Work out the finished part from the listing and answer in its coordinate system (mm). Face numbers are marked on the shaded views. A direction names the side the tool comes from. Give positions to 0.01 mm unless a question says otherwise; leave off trailing zeros. Loops run counter-clockwise (first coordinate to the right, second up) from the corner with the lowest first, then second, coordinate; pieces in that order, holes last.
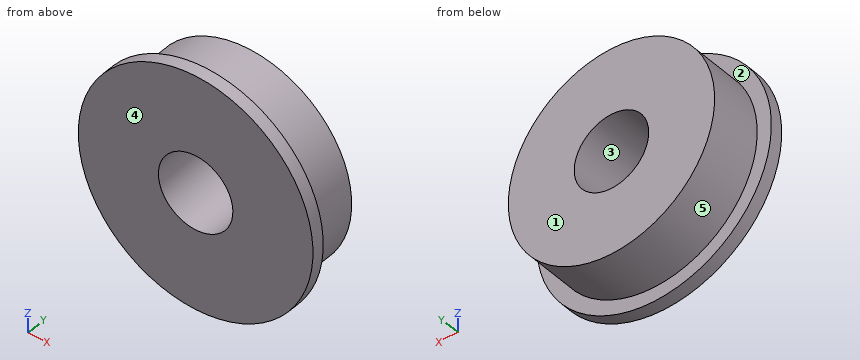
from build123d import *

# Parameters (mm, degrees)
SKETCH1_R           = 12.51
BOSS_EXTRUDE1_DEPTH = 1.36
BOSS_EXTRUDE2_START = -1.36
SKETCH2_R           = 11
BOSS_EXTRUDE2_DEPTH = 6.98
SKETCH3_R           = 3.97
CUT_EXTRUDE1_DEPTH  = 20.018953704


with BuildPart() as part:
    # Sketch1 → Boss-Extrude1 (new body)
    with BuildSketch(Plane(origin=(0, 0, 0), x_dir=(1, 0, 0), z_dir=(0, 1, 0))):
        with Locations(Location((0, 0, 0), (0, 0, 270))):
            Circle(SKETCH1_R)
    extrude(amount=BOSS_EXTRUDE1_DEPTH)

    # Sketch2 → Boss-Extrude2 (add)
    with BuildSketch(Plane(origin=(0, 1.36, 0), x_dir=(1, 0, 0), z_dir=(0, 1, 0)).offset(BOSS_EXTRUDE2_START)):
        with Locations(Location((0, 0, 0), (0, 0, 270))):
            Circle(SKETCH2_R)
    extrude(amount=BOSS_EXTRUDE2_DEPTH)

    # Sketch3 → Cut-Extrude1 (cut, through all)
    with BuildSketch(Plane(origin=(0, 6.98, 0), x_dir=(1, 0, 0), z_dir=(0, 1, 0))):
        with Locations(Location((0, 0, 0), (0, 0, 270))):
            Circle(SKETCH3_R)
    extrude(amount=-CUT_EXTRUDE1_DEPTH, mode=Mode.SUBTRACT)


solid = part.part
Item 1: Find section A-A, the plane x = 0. Write down the section's boundary in (y, z), plus the area to 3 significant figures.
Item 2: Flat-ended cylindrical pins translate along their axes: pin 1 Ø3 at (x, y) = (-3.5, 4) entering from -Z; pin 2 Ø1.5 at (y, z) = (4.5, -8) entering from +X; pin 3 Ø2 at (y, z) = (1, -6.5) entering from -X. Find the tip coordinate at first contact, or state that the pin passes through.
Item 3: Determine the mould class of the marked faces 3, 4 and 5 for opening direction Z: released by +Z, released by -Z, zero draft, split by the parting line, or undercut.
Item 4: Find section D-D, the plane z = -5.5. Write down the section's boundary in (x, y).
Item 5: Find section B-B, the plane z = 0. Write down the section's boundary in (x, y).
Item 6: Consider line 1 (X direction, y = 2, z = 0); line 2 (X direction, y = 6.75, z = 3.5). Determine where each line is inside the solid, lowest interval first.
Item 7: For the marked faces 1 and 2, determine the directions among +Z, -Z, +X, -X, +Y, -Y from which every point of the face is accessible in a straight line to the end or side of a thin tool.
Item 8: Find section C-C, the plane y = 6.25. Write down the section's boundary in (x, z), plus the area to 3 significant figures.
Ans:
1. outline: (0, -12.51) - (1.36, -12.51) - (1.36, -11) - (6.98, -11) - (6.98, -3.97) - (0, -3.97) - close; (0, 3.97) - (6.98, 3.97) - (6.98, 11) - (1.36, 11) - (1.36, 12.51) - (0, 12.51) - close
1. area: 102 mm2
2. pin 1: stops at z = -10.82
2. pin 2: stops at x = 8.27
2. pin 3: stops at x = -11.24
3. face 3: undercut
3. face 4: zero draft
3. face 5: split by the parting line
4. outline: (-11.24, 0) - (11.24, 0) - (11.24, 1.36) - (9.53, 1.36) - (9.53, 6.98) - (-9.53, 6.98) - (-9.53, 1.36) - (-11.24, 1.36) - close
5. outline: (-12.51, 0) - (-3.97, 0) - (-3.97, 6.98) - (-11, 6.98) - (-11, 1.36) - (-12.51, 1.36) - close; (3.97, 0) - (12.51, 0) - (12.51, 1.36) - (11, 1.36) - (11, 6.98) - (3.97, 6.98) - close
6. line 1: x = -11 to -3.97, 3.97 to 11
6. line 2: x = -10.43 to -1.87, 1.87 to 10.43
7. face 1: +Z, -Z, +X, -X, +Y
7. face 2: +Y
8. outline: circle Ø22 at (0, 0); hole circle Ø7.94 at (0, 0)
8. area: 331 mm2
